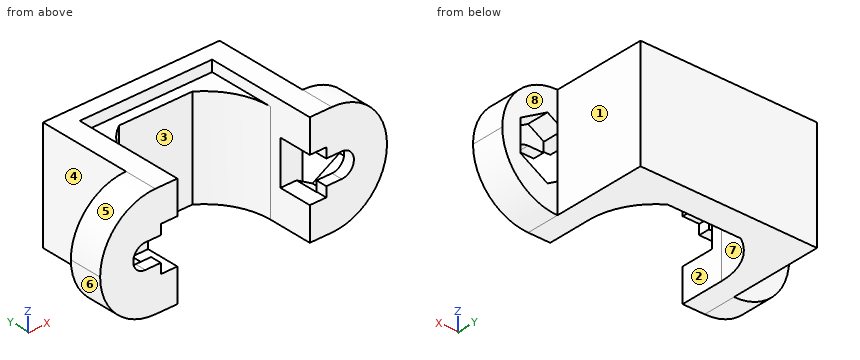
Autodesk Inventor part; units mm, degrees
ref_plane "YZ Plane" through (0, 0, 0) normal (1, 0, 0) x (0, 1, 0)
ref_plane "XZ Plane" through (0, 0, 0) normal (0, 1, 0) x (-1, 0, 0)
ref_plane "XY Plane" through (0, 0, 0) normal (0, 0, 1) x (1, 0, 0)
sketch "Эскиз1" plane through (0, 0, 0) normal (0, 0, 1) x (1, 0, 0)
  circle A0 centre (0, 0) radius 6
  line L0 (-6, 0) -> (6, 0)
  line L1 (6, 0) -> (6, 5)
  line L2 (6, 5) -> (-6, 5)
  line L3 (-6, 5) -> (-6, 0)
  line L4 (-6, 0) -> (6, 0)
  line L5 (6, 0) -> (6, -4)
  line L6 (6, -4) -> (-6, -4)
  line L7 (-6, -4) -> (-6, 0)
  line L8 (-6, -4) -> (-8, -4)
  line L9 (-8, -4) -> (-8, 5)
  line L10 (-8, 5) -> (-6, 5)
  line L11 (-6, 5) -> (-6, -4)
  line L12 (6, 5) -> (8, 5)
  line L13 (8, 5) -> (8, -4)
  line L14 (8, -4) -> (6, -4)
  line L15 (6, -4) -> (6, 5)
  line L16 (-8, 5) -> (8, 5)
  line L17 (8, 5) -> (8, 7.5)
  line L18 (8, 7.5) -> (-8, 7.5)
  line L19 (-8, 7.5) -> (-8, 5)
  line L20 (-8, -4) -> (-13, -4)
  line L21 (-13, -4) -> (-13, -1)
  line L22 (-13, -1) -> (-8, -1)
  line L23 (-8, -1) -> (-8, -4)
  line L24 (8, -4) -> (13, -4)
  line L25 (13, -4) -> (13, -1)
  line L26 (13, -1) -> (8, -1)
  line L27 (8, -1) -> (8, -4)
  point P0 (8, -1)
  point P1 (-8, -1)
  point P2 (-3.3166, 5)
  point P3 (3.3166, 5)
  dimension "d0" = 12
  dimension "d1" = 5
  dimension "d2" = 4
  dimension "d3" = 2
  dimension "d4" = 2
  dimension "d5" = 2.5
  dimension "d8" = 5
  dimension "d9" = 5
  dimension "d37" = 3
extrude "Выдавливание1" add sketch "Эскиз1" along normal blind 10 contours A0 L2 L1 | L1 L12 L13 L14 L5 | L2 A0 | A0 L2 L10 L19 L18 L17 L12 | L3 L2 A0 | L7 L8 L9 L10 L3 | L13 L26 L25 L24 | L20 L21 L22 L9
sketch "Эскиз2" plane through (-13, -1, 0) normal (0, 1, 0) x (1, 0, 0)
  line L0 (5, 0) -> (0, 0)
  line L1 (2.5, 0) -> (2.5, -10)
  line L2 (5, -10) -> (0, -10)
  line L3 (26, -10) -> (21, -10)
  line L4 (23.5, -10) -> (23.5, 0)
  line L5 (26, 0) -> (21, 0)
  line L6 (23.5, -5) -> (21.9, -5)
  line L7 (2.5, -5) -> (4.1, -5)
  point P0 (13, 0)
  dimension "d17" = 1.6
  dimension "d18" = 1.6
hole "Отверстие2" at (-8.9, -1, 5) at (8.9, -1, 5) direction (0, -1, 0) diameter 2.2 end through all
sketch "Эскиз3" plane through (8, -1, 0) normal (0, 1, 0) x (1, 0, 0)
  arc A0 (-16, -4.3675) -> (-16, -5.6325) centre (-16.9, -5) ccw
  arc A1 (0, -5.6325) -> (0, -4.3675) centre (0.9, -5) ccw
  line L0 (3.35, -6.4145) -> (0.9, -7.829)
  line L1 (0.9, -7.829) -> (-1.55, -6.4145)
  line L2 (-1.55, -6.4145) -> (-1.55, -3.5855)
  line L3 (-1.55, -3.5855) -> (0.9, -2.171)
  line L4 (0.9, -2.171) -> (3.35, -3.5855)
  line L5 (3.35, -3.5855) -> (3.35, -6.4145)
  line L6 (-19.35, -3.5855) -> (-16.9, -2.171)
  line L7 (-16.9, -2.171) -> (-14.45, -3.5855)
  line L8 (-14.45, -3.5855) -> (-14.45, -6.4145)
  line L9 (-14.45, -6.4145) -> (-16.9, -7.829)
  line L10 (-16.9, -7.829) -> (-19.35, -6.4145)
  line L11 (-19.35, -6.4145) -> (-19.35, -3.5855)
  line L12 (-21, 0) -> (-21, -10)
  line L13 (5, 0) -> (5, -10)
  point P0 (-8, 0)
  dimension "d26" = 4.9
extrude "Выдавливание2" cut sketch "Эскиз3" against normal blind 2
fillet "Сопряжение1" radius 5 4 edges at (-13, -2.5, 0) (-13, -2.5, 10) (13, -2.5, 0) (13, -2.5, 10)
sketch "Эскиз5" plane through (0, 0, 10) normal (0, 0, 1) x (1, 0, 0)
  line L0 (-6, -4) -> (-6, 0)
  line L1 (-6, 0) -> (6, 0)
  line L2 (6, 0) -> (6, 6)
  line L3 (6, 6) -> (-6, 6)
  line L4 (-6, 6) -> (-6, 0)
  line L5 (6, 0) -> (6, -4)
  line L6 (-3.3166, 5) -> (3.3166, 5)
  point P0 (0, 0)
  dimension "d34" = 1
extrude "Выдавливание4" cut sketch "Эскиз5" against normal blind 1
sketch "Эскиз6" plane through (-6, -4, 0) normal (0, -1, 0) x (1, 0, 0)
  line L0 (-1.5, 7) -> (0, 7)
  line L1 (0, 7) -> (0, 3)
  line L2 (0, 3) -> (-1.5, 3)
  line L3 (-1.5, 3) -> (-1.5, 7)
  line L4 (0, 0) -> (0, 10)
  line L5 (-2.9, 3.9) -> (-1.5, 3.9)
  line L6 (-1.5, 3.9) -> (-1.5, 6.1)
  line L7 (-1.5, 6.1) -> (-2.9, 6.1)
  line L8 (-2.9, 6.1) -> (-2.9, 3.9)
  circle A0 centre (-2.9, 5) radius 1.1
  line L9 (14, 0) -> (-2, 0)
  line L10 (6, 0) -> (6, 10)
  line L11 (0, 10) -> (12, 10)
  line L12 (13.5, 7) -> (12, 7)
  line L13 (12, 7) -> (12, 3)
  line L14 (12, 3) -> (13.5, 3)
  line L15 (13.5, 3) -> (13.5, 7)
  line L16 (14.9, 3.9) -> (13.5, 3.9)
  line L17 (13.5, 3.9) -> (13.5, 6.1)
  line L18 (13.5, 6.1) -> (14.9, 6.1)
  line L19 (14.9, 6.1) -> (14.9, 3.9)
  point P0 (0, 5)
  point P1 (-2.9, 3.9)
  point P2 (-2.9, 6.1)
  point P3 (-2.9, 3.9)
  point P4 (-2.9, 6.1)
  point P5 (12, 5)
  point P6 (14.9, 5)
  point P7 (14.9, 5)
  dimension "d38" = 4
  dimension "d42" = 1.5
extrude "Выдавливание5" cut sketch "Эскиз6" against normal up to surface (3 mm away) contours L0 L1 L2 L3 | L3 L5 A0 L7 | A0 L8 | L15 L14 L13 L12 | L18 L19 L16 L15 picked at (-2.5898, 5.2959)
properties part number "Кронштейн для двигателей серии N"
Work out the finished part from the listing and answer in its coordinate system (mm). Face numbers are marked on the shaded views. A direction names the side the tool comes from. Round coordinates to 2 decimals unless told otherwise and drop trailing zeros. Loops run counter-clockwise (first coordinate to the right, second up) from the corner with the lowest first, then second, coordinate; pieces in that order, holes last. Notation, with made-up numbers: M 40,64.5 L 71,64.5 A20 cw 71,93.5 Z; hole C 31.25,-12 d6. An arc over 180 degrees is marked long. Use CSV: the item, a comma, the result in double quotes.
Q1. Section B-B, the plane x = -8.5 is taken. Determine the outline of the cut face in (y, z).
Determined:
outline,"M -4,0.03 L -1,0.03 L -1,2.4 L -3,2.4 L -3,3.9 L -4,3.9 Z; M -4,6.1 L -3,6.1 L -3,7.6 L -1,7.6 L -1,9.97 L -4,9.97 Z"
Q2. Section C-C, the plane x = 1.75 is taken. Determine the outline of the cut face in (y, z), then the cut area to 3 significant figures.
Determined:
outline,"M 5,0 L 7.5,0 L 7.5,10 L 6,10 L 6,9 L 5,9 Z"
area,"24.0 mm2"
Q3. A tool of negligible diameter and unlimited length cuts with its end or side. For the marked faces 1, 2, 3, 4 and 5, from which of +Z, -Z, +X, -X, +Y, -Y can it reach the whole face along a straight path? Write none if from no direction.
Determined:
face 1,"+Z, -Z, +X, +Y"
face 2,"+Z, -Y"
face 3,"+Z, -Z, -Y"
face 4,"+Z, -Z, -X, +Y"
face 5,"+Z, -X, +Y, -Y"
Q4. Each of these flat-tipped pins is pushed along its axis until it touches: pin 1 (0.6 mm diameter, centred on y = -1.5, z = 5.5, fed in from +X); pin 2 (1.8 mm diameter, centred on x = 0, y = 4.5, fed in from +Z); pin 3 (3 mm diameter, centred on y = 1.5, z = 6, fed in from -X). Where does it stop, or does it pass through?
Determined:
pin 1,"x = 13"
pin 2,"z = 9"
pin 3,"x = -8"
Q5. Consider L1, parallel to Y at x = 1.25, z = 2; L2, parallel to Y at x = -7.75, z = 5.25; L3, parallel to Z at x = -10.75, y = -1.25. Determine where each line is inside the solid, lowest interval first.
Determined:
L1,"5 to 7.5"
L2,"-1 to 7.5"
L3,"0.82 to 3.24, 6.76 to 9.18"
Q6. Section D-D, the plane z = 5.5 is taken. Determine the outline of the cut face in (x, y), then the cut area to 3 significant figures.
Determined:
outline,"M -12.97,-4 L -9.88,-4 L -9.88,-3 L -11.35,-3 L -11.35,-1 L -12.97,-1 Z; M -8,-1 L -6,-1 L -6,0 A6 cw -3.32,5 L 3.32,5 A6 cw 6,0 L 6,-1 L 8,-1 L 8,7.5 L -8,7.5 Z; M 9.88,-4 L 12.97,-4 L 12.97,-1 L 11.35,-1 L 11.35,-3 L 9.88,-3 Z"
area,"84.6 mm2"
Q7. The mould has two halves that part along X. Classify the marked faces 6, 7 and 8: pulls with the +X half, pulls with the -X half, needs draft (parallel to the pull), parting line crosses it, or undercut.
Determined:
face 6,"pulls with the -X half"
face 7,"undercut"
face 8,"needs draft"
